Input: part model. Units: mm. Frame: model coordinates. A direction names the side the tool comes from. Coordinates: 2 decimals unless noted, no trailing zeros. Loops run counter-clockwise (first coordinate to the right, second up) from the corner with the lowest first, then second, coordinate; pieces in that order, holes last.
Item 1: Section C-C on y = -3.75. Return loops of the section in (x, z), and give its area (3 significant figures).
Item 2: Contact query for flat-ended pins moving along their axis: P1, Ø2, axis at x = -6.5, z = 1.5, coming from the +Y side; P2, Ø2, axis at x = -37, y = -3, coming from the +Z side; P3, Ø2, axis at y = 4.5, z = 4, coming from the +X side; P4, Ø1.7, axis at x = -21.5, y = 10, coming from the +Z side. Output: stop coordinate, or through.
Item 3: Reachability of faces 1 (the flat face through (-6.3, -3.9, 3.4)), 2 (the flat face through (-22, -0.4, 2)), 3 (the flat face through (-34, 6, 4)) from +Z, -Z, +X, -X, +Y, -Y: full face, straight path, thin tool, end or side. Return the list, or none.
Item 4: Section A-A on x = -4.5. Return loops of the section in (y, z), and give its area (3 significant figures).
Item 5: Section B-B on y = 10. Return loops of the section in (x, z).
Item 6: Ray query, line 1 along X through (y, z) = (-3.75, 1.35); line 2 along X through (y, z) = (10, 4.15); line 3 along Y through (x, z) = (-38.5, 1.4). Return the intervals inside material, ascending.
Item 7: Pull-direction query (Y, two-part tool) for faces 4 (the flat face through (-36.8, -3.9, 3.4)), 5 (the cylindrical face through (-20.133, 10.303, 4.386)), 6 (the flat face through (-22, -7.5, 2)); classes: released by +Y, released by -Y, zero draft, split by the parting line, or undercut.
Item 8: Section D-D on x = -21.5. Return loops of the section in (y, z), and give its area (3 significant figures).
Autodesk Inventor part; units mm, degrees
ref_plane "YZ Plane" through (0, 0, 0) normal (1, 0, 0) x (0, 1, 0)
ref_plane "XZ Plane" through (0, 0, 0) normal (0, 1, 0) x (-1, 0, 0)
ref_plane "XY Plane" through (0, 0, 0) normal (0, 0, 1) x (1, 0, 0)
sketch "Sketch1" plane through (0, 0, 0) normal (0, 0, 1) x (1, 0, 0)
  line L0 (0, 0) -> (-43, 0)
  line L1 (-43, 0) -> (-43, -7.5)
  line L2 (-43, -7.5) -> (0, -7.5)
  line L3 (0, -7.5) -> (0, 0)
  dimension "d0" = 43
  dimension "d1" = 7.5
extrude "Extrusion1" add sketch "Sketch1" along normal blind 3.4
sketch "Sketch3" plane through (0, 0, 3.4) normal (0, 0, 1) x (1, 0, 0)
  circle A0 centre (-38.5, -3.75) radius 1.5
  circle A1 centre (-4.5, -3.75) radius 1.5
  point P0 (0, 0)
  dimension "d4" = 3
  dimension "d5" = 3
hole "Hole1" at (-38.5, -3.75, 3.4) at (-4.5, -3.75, 3.4) direction (0, 0, -1) diameter 2.8 end through all
sketch "Sketch4" plane through (0, 0, 3.4) normal (0, 0, 1) x (1, 0, 0)
  line L0 (-43, 0) -> (-43, -7.5)
  line L1 (-43, 0) -> (-34, 0)
  line L2 (-34, 0) -> (-34, -3.75)
  line L3 (-34, -3.75) -> (-43, -3.75)
  line L4 (-43, -3.75) -> (-43, 0)
  line L5 (0, 0) -> (-9, 0)
  line L6 (-9, 0) -> (-9, -3.75)
  line L7 (-9, -3.75) -> (0, -3.75)
  line L8 (0, -3.75) -> (0, 0)
  line L9 (-9, 0) -> (-34, 0)
  line L10 (-34, 0) -> (-34, -2)
  line L11 (-34, -2) -> (-9, -2)
  line L12 (-9, -2) -> (-9, 0)
  dimension "d13" = 9
  dimension "d14" = 9
  dimension "d15" = 2
extrude "Extrusion2" add sketch "Sketch4" along normal blind 2 contours L9 L6 L11 L2
sketch "Sketch5" plane through (-43, 0, 0) normal (0, 1, 0) x (1, 0, 0)
  line L0 (43, -3.4) -> (34, -3.4)
  line L1 (9, -5.4) -> (34, -5.4)
  line L2 (34, -3.4) -> (9, -3.4)
  line L3 (9, -3.4) -> (9, -5.4)
  line L4 (9, -5.4) -> (34, -5.4)
  line L5 (34, -5.4) -> (34, -3.4)
  point P0 (43, 0)
extrude "Extrusion3" add sketch "Sketch5" along normal blind 20 and the other way blind 7.5
sketch "Sketch6" plane through (-43, 0, 0) normal (0, 1, 0) x (1, 0, 0)
  line L0 (43, 0) -> (43, -3.4)
  line L1 (0, 0) -> (0, -3.4)
  line L2 (43, 0) -> (0, 0)
  line L3 (0, 0) -> (0, -3.4)
  line L4 (0, -3.4) -> (43, -3.4)
  line L5 (43, -3.4) -> (43, 0)
  dimension "d22" = 43
extrude "Extrusion4" cut sketch "Sketch6" against normal blind 0.4
fillet "Fillet3" radius 2 1 edges at (-43, -3.95, 3.4)
fillet "Fillet4" radius 2 1 edges at (0, -3.95, 3.4)
sketch "Sketch7" plane through (0, 0, 5.4) normal (0, 0, 1) x (1, 0, 0)
  line L0 (-9, -7.5) -> (-34, -7.5)
  line L1 (-9, -7.5) -> (-21.5, -7.5)
  line L2 (-21.5, -7.5) -> (-21.5, 0)
  line L3 (-21.5, 0) -> (-9, 0)
  line L4 (-9, 0) -> (-9, -7.5)
  line L5 (-21.5, 0) -> (-21.5, 10)
  circle A0 centre (-21.5, 10) radius 1.4
  point P0 (0, 0)
  dimension "d32" = 12.5
  dimension "d33" = 7.5
  dimension "d34" = 10
  dimension "d35" = 2.8
hole "Hole2" at (-21.5, 10, 5.4) direction (0, 0, -1) diameter 2.8 end through all
properties part number "Enclosure clip simple"
Results found:
1. outline: (-43, 0) - (-39.9, 0) - (-39.9, 3.4) - (-41, 3.4) arc R2 ccw to (-43, 1.4) - close; (-37.1, 0) - (-5.9, 0) - (-5.9, 3.4) - (-9, 3.4) - (-9, 5.4) - (-34, 5.4) - (-34, 3.4) - (-37.1, 3.4) - close; (-3.1, 0) - (0, 0) - (0, 1.4) arc R2 ccw to (-2, 3.4) - (-3.1, 3.4) - close
1. area: 175 mm2
2. P1: stops at y = -0.4
2. P2: stops at z = 3.4
2. P3: stops at x = -9
2. P4: passes through
3. face 1: +Z, +X, +Y, -Y
3. face 2: -Z, +X, -X, +Y
3. face 3: +Z, -X, +Y, -Y
4. outline: (-7.5, 0) - (-5.15, 0) - (-5.15, 3.4) - (-7.5, 3.4) - close; (-2.35, 0) - (-0.4, 0) - (-0.4, 3.4) - (-2.35, 3.4) - close
4. area: 14.6 mm2
5. outline: (-34, 3.4) - (-22.9, 3.4) - (-22.9, 5.4) - (-34, 5.4) - close; (-20.1, 3.4) - (-9, 3.4) - (-9, 5.4) - (-20.1, 5.4) - close
6. line 1: x = -43 to -39.9, -37.1 to -5.9, -3.1 to 0
6. line 2: x = -34 to -22.9, -20.1 to -9
6. line 3: y = -7.5 to -5.15, -2.35 to -0.4
7. face 4: zero draft
7. face 5: undercut
7. face 6: released by -Y
8. outline: (-7.5, 0) - (-0.4, 0) - (-0.4, 3.4) - (8.6, 3.4) - (8.6, 5.4) - (-7.5, 5.4) - close; (11.4, 3.4) - (20, 3.4) - (20, 5.4) - (11.4, 5.4) - close
8. area: 73.5 mm2
